Autodesk Inventor part; units mm, degrees
ref_plane "YZ Plane" through (0, 0, 0) normal (1, 0, 0) x (0, 1, 0)
ref_plane "XZ Plane" through (0, 0, 0) normal (0, 1, 0) x (-1, 0, 0)
ref_plane "XY Plane" through (0, 0, 0) normal (0, 0, 1) x (1, 0, 0)
sketch "Sketch1" plane through (0, 0, 0) normal (0, 1, 0) x (-1, 0, 0)
  line L0 (-8.255, -31.4325) -> (8.255, -31.4325)
  line L1 (20.955, -18.7325) -> (20.955, 31.4325)
  line L2 (20.955, 31.4325) -> (-20.955, 31.4325)
  line L3 (-20.955, 31.4325) -> (-20.955, -18.7325)
  line L4 (-20.955, -31.4325) -> (20.955, 31.4325) construction
  line L5 (20.955, -31.4325) -> (-20.955, 31.4325) construction
  arc A0 (8.255, -31.4325) -> (20.955, -18.7325) centre (8.255, -18.7325) ccw
  arc A1 (-20.955, -18.7325) -> (-8.255, -31.4325) centre (-8.255, -18.7325) ccw
  point P0 (0, 0)
  dimension "d0" = 62.865
  dimension "d1" = 41.91
  dimension "d2" = 12.7
extrude "Extrusion1" add sketch "Sketch1" along normal blind 12.7
properties part number "Fixture_Airpot_Support_2"
For this review, take the finished solid that the model builds, in its own axes (mm). Give positions to 0.01 mm unless a question says otherwise; leave off trailing zeros. Order: outer loops, then holes, each group sorted by start corner. A loop starts at its lowest first (then second) coordinate and runs counter-clockwise, first axis right, second up. Notation, with made-up numbers: (-8.75, -5.75) - (45.25, -5.75) arc R19 ccw to (45.25, -0.75) - close; hole circle Ø5 at (11.5, 22). An arc over 180 degrees is marked (long way). Answer as a JSON object with one key per item and string values. Group by question number.
Item 1: Take a section at C-C on x = -16. Give the boundary of the cut face in (y, z).
Item 2: Take a section at A-A on y = 2.5. Give the boundary of the cut face in (x, z) (1 decimal), and give its area (3 significant figures).
Item 3: Take a section at B-B on z = -25.5. Give the boundary of the cut face in (x, y), and give its area (3 significant figures).
Item 4: Clearance check with a flat-ended pin moving along its axis: pin 1 Ø1 at (y, z) = (7.5, -21.5) entering from -X. State where the tip first meets the part, or that it passes through.
Item 5: Wall thickness on line 1 along Z through (x, y) = (-8.5, 1); line 2 along Z through (x, y) = (15, 10); line 3 along X through (y, z) = (8.5, -22): over which ranges is each line inside the solid? List them lowest first.
Reported:
{
 "1": {"outline": "(0, -28.8) - (12.7, -28.8) - (12.7, 31.43) - (0, 31.43) - close"},
 "2": {"outline": "(-21, -18.7) arc R12.7 ccw to (-8.3, -31.4) - (8.3, -31.4) arc R12.7 ccw to (21, -18.7) - (21, 31.4) - (-21, 31.4) - close", "area": "2,570 mm^2"},
 "3": {"outline": "(-19, 0) - (19, 0) - (19, 12.7) - (-19, 12.7) - close", "area": "483 mm^2"},
 "4": {"pin 1": "x = -20.75"},
 "5": {"line 1": "-31.43 to 31.43", "line 2": "-29.49 to 31.43", "line 3": "-20.53 to 20.53"}
}
